Source: CAD feature listing. Evaluate the final solid. Frame: model axes, mm. Round coordinates to 2 decimals unless told otherwise and drop trailing zeros. Write each loop counter-clockwise with the first axis right and the second up, starting at its lowest first coordinate (ties: lowest second). Pieces come first, ordered by that corner, then holes. Notation, with made-up numbers: (19, 58) -> (52, 58) arc R29 cw to (52, 78) -> close; hole circle Ø9 at (16, 59.25). An arc over 180 degrees is marked (long way). Return JSON: item names as keys, results as strings. Group by question number.
from build123d import *

# Parameters (mm, degrees)
SKETCH1_W           = 5
SKETCH1_H           = 10
BOSS_EXTRUDE1_DEPTH = 2.5
FILLET1_R           = 10
CUT_EXTRUDE1_REACH  = 125.085
SKETCH2_R           = 4.25


with BuildPart() as part:
    # Sketch1 → Boss-Extrude1 (new, symmetric)
    with BuildSketch(Plane(origin=(0, 0, 0), x_dir=(0, 1, 0), z_dir=(0, 0, 1))):
        Polygon((-55, 50), (-25, 20), (-25, -25), (25, -25), (25, 30), (20, 30), (20, 40), (25, 40), (25, 50), (-20, 50), (-20, 80), (-25, 80), (-25, 90), (-20, 90), (-20, 110), (-55, 110), align=None)
        with Locations((-22.5, 35)):
            Rectangle(SKETCH1_W, SKETCH1_H, mode=Mode.SUBTRACT)
    extrude(amount=BOSS_EXTRUDE1_DEPTH, both=True)

    # Fillet1
    fillet1_edges = [part.edges().sort_by_distance(p)[0] for p in [
        (-50, -55, 0),
        (-110, -55, 0),
        (25, 25, 0),
        (25, -25, 0),
        (-20, -25, 0),
    ]]
    fillet(fillet1_edges, radius=FILLET1_R)

    # Sketch2 → Cut-Extrude1 (cut, up to next)
    with BuildSketch(Plane.XY.offset(2.5), mode=Mode.PRIVATE) as cut_extrude1_sk1:
        with Locations((-95, -40)):
            Circle(SKETCH2_R)
    cut_extrude1_tool1 = extrude(cut_extrude1_sk1.sketch, amount=-CUT_EXTRUDE1_REACH, mode=Mode.PRIVATE) & part.part
    # Sketch2 → Cut-Extrude1 (cut, up to next)
    with BuildSketch(Plane.XY.offset(2.5), mode=Mode.PRIVATE) as cut_extrude1_sk2:
        with Locations((-55, -40)):
            Circle(SKETCH2_R)
    cut_extrude1_tool2 = extrude(cut_extrude1_sk2.sketch, amount=-CUT_EXTRUDE1_REACH, mode=Mode.PRIVATE) & part.part
    # Sketch2 → Cut-Extrude1 (cut, up to next)
    with BuildSketch(Plane.XY.offset(2.5), mode=Mode.PRIVATE) as cut_extrude1_sk3:
        with Locations((-5, 0)):
            Circle(SKETCH2_R)
    cut_extrude1_tool3 = extrude(cut_extrude1_sk3.sketch, amount=-CUT_EXTRUDE1_REACH, mode=Mode.PRIVATE) & part.part
    add(cut_extrude1_tool1.solids().sort_by_distance((-95, -40, 2.5))[0], mode=Mode.SUBTRACT)
    add(cut_extrude1_tool2.solids().sort_by_distance((-55, -40, 2.5))[0], mode=Mode.SUBTRACT)
    add(cut_extrude1_tool3.solids().sort_by_distance((-5, 0, 2.5))[0], mode=Mode.SUBTRACT)


solid = part.part
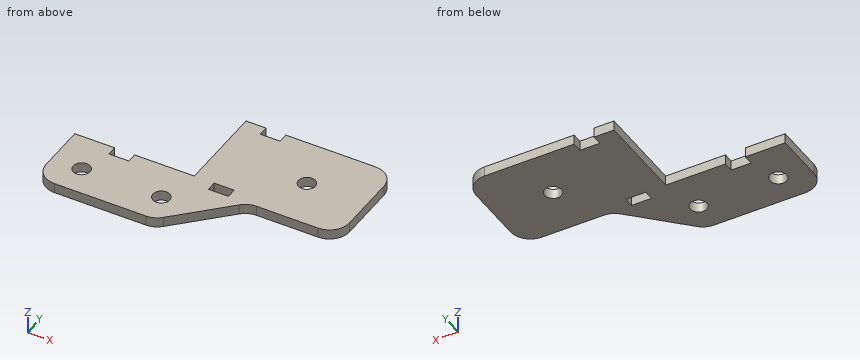
Item 1: First-contact query: pin 1 Ø2.5 at (y, z) = (22, 0.5) entering from +X; pin 2 Ø2.5 at (x, z) = (-7.5, 0) entering from -Y; pin 3 Ø2.5 at (x, z) = (-35, -1) entering from +Y; pin 4 Ø5 at (x, y) = (-55, -40) entering from -Z. Flat tips, straight axial feed; report the tip coordinate or a pass-through.
Item 2: Cut plane D-D on y = -40. Output: boundary loops of the cut face in (x, z), and give its area (3 significant figures).
Item 3: Cut plane A-A on x = -5. Output: boundary loops of the cut face in (y, z), and give its area (4 significant figures).
Item 4: Material intervals for probe 1 along Y at (x, z) = (-55, -0.4); probe 2 along Y at (x, z) = (-5, -1.7); probe 3 along X at (y, z) = (-20.5, 0.1), sorted ascending.
Item 5: Cut plane B-B on y = 0. Output: boundary loops of the cut face in (x, z), and give its area (4 significant figures).
Item 6: Cut plane C-C on z = 1.5. Output: boundary loops of the cut face in (x, y).
Here are the results:
{
 "1": {"pin 1": "stops at x = 23.18", "pin 2": "stops at y = -25", "pin 3": "stops at y = 20", "pin 4": "passes through"},
 "2": {"outline": "(-110, -2.5) -> (-99.25, -2.5) -> (-99.25, 2.5) -> (-110, 2.5) -> close; (-90.75, -2.5) -> (-59.25, -2.5) -> (-59.25, 2.5) -> (-90.75, 2.5) -> close; (-50.75, -2.5) -> (-35, -2.5) -> (-35, 2.5) -> (-50.75, 2.5) -> close", "area": "290 mm^2"},
 "3": {"outline": "(-25, -2.5) -> (-4.25, -2.5) -> (-4.25, 2.5) -> (-25, 2.5) -> close; (4.25, -2.5) -> (25, -2.5) -> (25, 2.5) -> (4.25, 2.5) -> close", "area": "207.5 mm^2"},
 "4": {"probe 1": "y = -55 to -44.25, -35.75 to -20", "probe 2": "y = -25 to -4.25, 4.25 to 25", "probe 3": "x = -110 to -90, -80 to -40, -30 to 23.35"},
 "5": {"outline": "(-50, -2.5) -> (-9.25, -2.5) -> (-9.25, 2.5) -> (-50, 2.5) -> close; (-0.75, -2.5) -> (25, -2.5) -> (25, 2.5) -> (-0.75, 2.5) -> close", "area": "332.5 mm^2"},
 "6": {"outline": "(-110, -45) arc R10 ccw to (-100, -55) -> (-54.14, -55) arc R10 ccw to (-47.07, -52.07) -> (-22.93, -27.93) arc R10 cw to (-15.86, -25) -> (15, -25) arc R10 ccw to (25, -15) -> (25, 15) arc R10 ccw to (15, 25) -> (-30, 25) -> (-30, 20) -> (-40, 20) -> (-40, 25) -> (-50, 25) -> (-50, -20) -> (-80, -20) -> (-80, -25) -> (-90, -25) -> (-90, -20) -> (-110, -20) -> close; hole circle Ø8.5 at (-95, -40); hole circle Ø8.5 at (-55, -40); hole (-40, -25) -> (-30, -25) -> (-30, -20) -> (-40, -20) -> close; hole circle Ø8.5 at (-5, 0)"}
}
